Geometry check sheet. Reference: drawing and pictorial views, mm from the part's lowest x, y, z. A direction names the side the tool comes from. Round coordinates to 2 decimals unless told otherwise and drop trailing zeros. Loops run counter-clockwise (first coordinate to the right, second up) from the corner with the lowest first, then second, coordinate; pieces in that order, holes last. Notation, with made-up numbers: (0, -27) - (26, -27) arc R21 cw to (26, -20) - close; hole circle Ø8 at (22, 73.5). An arc over 180 degrees is marked (long way). Return JSON: item names as keys, results as strings.
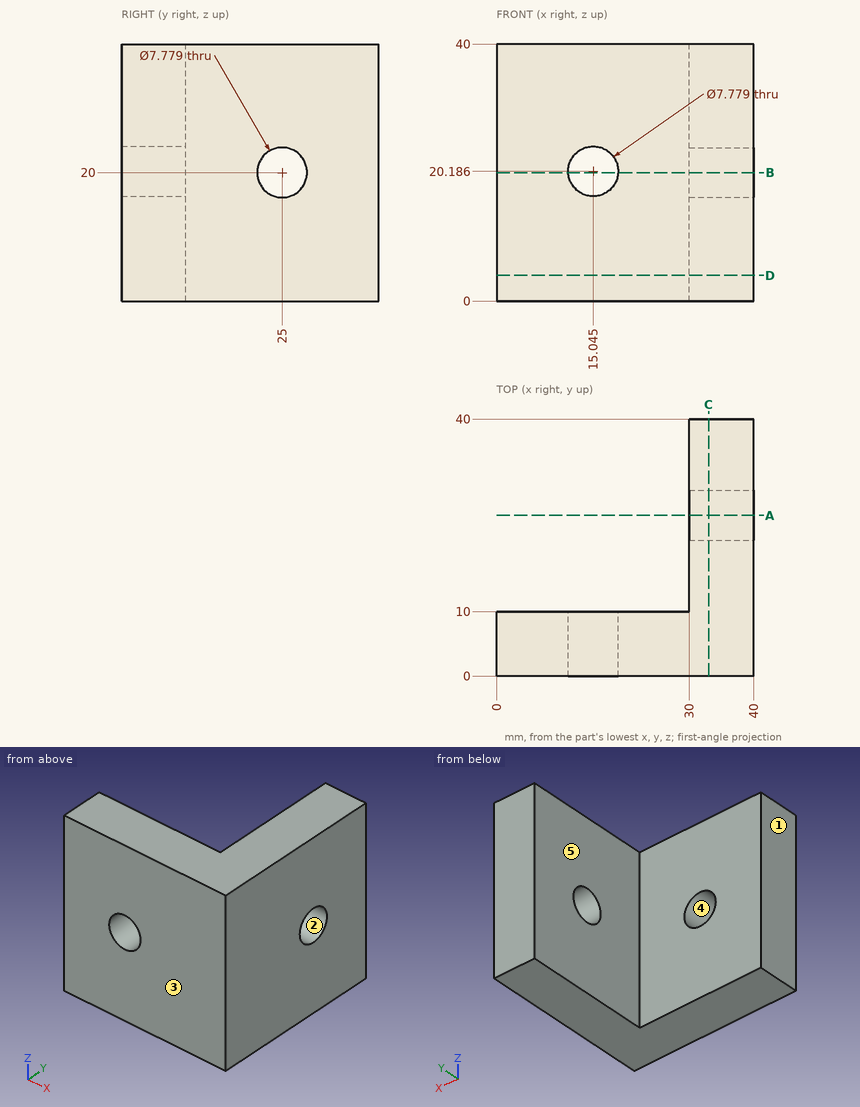
Q1. Depth check by flat-ended pin: P1, Ø8, axis at x = 5.5, y = 11, coming from the +Z side; P2, Ø10, axis at x = 15.05, z = 20.19, coming from the +Y side; P3, Ø9, axis at y = 25, z = 20, coming from the -X side. Enter the tip coordinate at first touch or a pass-through.
Answer key:
{"P1": "stops at z = 40", "P2": "stops at y = 10", "P3": "stops at x = 30"}
Q2. Draft check along Y on the marked faces 1, 2 and 3. Enter one of: released by +Y, released by -Y, zero draft, split by the parting line, or undercut.
Answer key:
{"face 1": "zero draft", "face 2": "undercut", "face 3": "released by -Y"}
Q3. Sectioned sample at A-A (y = 25). Enter the section's corners in (x, z), plus the area to 3 significant figures.
Answer key:
{"outline": "(30, 0) - (40, 0) - (40, 16.11) - (30, 16.11) - close; (30, 23.89) - (40, 23.89) - (40, 40) - (30, 40) - close", "area": "322 mm²"}
Q4. Tool access check on the marked faces 4 and 5. Record the directions out of +Z, -Z, +X, -X, +Y, -Y that give a thin tool (end or side, any length) a straight path to the whole face; none if there is none.
Answer key:
{"face 4": "+Y, -Y", "face 5": "+Z, -Z, -X, +Y"}
Q5. Sectioned sample at B-B (z = 20). Enter the section's corners in (x, y).
Answer key:
{"outline": "(0, 0) - (11.16, 0) - (11.16, 10) - (0, 10) - close; (18.93, 0) - (40, 0) - (40, 21.11) - (30, 21.11) - (30, 10) - (18.93, 10) - close; (30, 28.89) - (40, 28.89) - (40, 40) - (30, 40) - close"}
Q6. Sectioned sample at D-D (z = 4). Enter the section's corners in (x, y), plus the area to 3 significant figures.
Answer key:
{"outline": "(0, 0) - (40, 0) - (40, 40) - (30, 40) - (30, 10) - (0, 10) - close", "area": "700 mm²"}
Q7. Sectioned sample at C-C (x = 33). Enter the section's corners in (y, z), plus the area to 3 significant figures.
Answer key:
{"outline": "(0, 0) - (40, 0) - (40, 40) - (0, 40) - close; hole circle Ø7.78 at (25, 20)", "area": "1,550 mm²"}
Q8. Scan lines: probe 1 along Z at (x, y) = (38, 25); probe 2 along Y at (x, z) = (32, 20); probe 3 along X at (y, z) = (31.5, 10.5). Record each from-to range of solid material in increasing order. Write a range as [from, to].
Answer key:
{"probe 1": "z = [0, 16.11], [23.89, 40]", "probe 2": "y = [0, 21.11], [28.89, 40]", "probe 3": "x = [30, 40]"}
